Autodesk Inventor part; units mm, degrees
ref_plane "YZ Plane" through (0, 0, 0) normal (1, 0, 0) x (0, 1, 0)
ref_plane "XZ Plane" through (0, 0, 0) normal (0, 1, 0) x (-1, 0, 0)
ref_plane "XY Plane" through (0, 0, 0) normal (0, 0, 1) x (1, 0, 0)
sketch "Эскиз1" plane through (0, 0, 0) normal (0, 1, 0) x (-1, 0, 0)
  circle A0 centre (0, 0) radius 106.25
  arc A1 (-95.3337, -46.91) -> (-95.3337, 46.91) centre (-154.2365, 0) ccw
  arc A2 (95.3337, 46.91) -> (95.3337, -46.91) centre (154.2365, 0) ccw
  line L0 (-154.2365, 0) -> (154.2365, 0)
  line L1 (-95.3337, 46.91) -> (-55.3337, 46.91) construction
  line L2 (95.3337, 46.91) -> (55.3337, 46.91) construction
  point P0 (74.5593, -32.2924)
  dimension "d5" = 212.5
  dimension "d16" = 75.3
  dimension "d17" = 75.3
  dimension "d18" = 93.82
  dimension "d19" = 40
  dimension "d20" = 93.82
sketch "Эскиз2" plane through (0, 0, 0) normal (0, 0, 1) x (1, 0, 0)
  line L0 (106.25, 0) -> (-106.25, 0)
  line L1 (106.25, 0) -> (106.25, -70.1)
  line L2 (106.25, -9.1) -> (108.25, -9.1) construction
  line L3 (-149.15, 0) -> (151.15, 0)
  line L4 (106.25, -70.1) -> (104.25, -70.1)
  line L5 (104.25, -70.1) -> (104.25, -10.7208)
  line L6 (106.25, -9.1) -> (58.25, 0)
  line L7 (104.25, -10.7208) -> (58.25, -2)
  line L8 (58.25, -2) -> (58.25, 0) construction
  line L9 (50.25, 0) -> (58.25, 0)
  line L10 (50.25, 0) -> (50.25, -2)
  line L11 (50.25, -2) -> (58.25, -2)
  line L12 (0, -84.12) -> (0, 14.02)
  point P0 (0, 0)
  dimension "d0" = 70.1
  dimension "d1" = 61
  dimension "d7" = 2
  dimension "d10" = 50.25
  dimension "d11" = 8
  dimension "d34" = 2
  dimension "d35" = 1.965
revolve "Вращение1" add sketch "Эскиз2" angle 360 about axis through (0, -10, 0) along (0, 1, 0) contours L6 L1 L4 L5 L7 L11 L10 L0
chamfer "Фаска1" distance 2.5 angle 45 1 edges at (-104.25, -10.7208, 0)
extrude "Выдавливание1" cut sketch "Эскиз1" against normal through all contours L0 A2 A0 | A0 A2 L0 | A1 L0 A0 | A0 L0 A1
sketch "Эскиз3" plane through (0, 0, 0) normal (0, 1, 0) x (1, 0, 0)
  line L0 (148.75, 0) -> (-148.75, 0) construction
  line L1 (0, 148.75) -> (0, -148.75) construction
  circle A0 centre (0, 0) radius 50.25
  circle A1 centre (0, 0) radius 58.25
  circle A2 centre (0, 0) radius 54.25 construction
  circle A3 centre (-54.25, 0) radius 1.65
  circle A4 centre (0, 54.25) radius 1.65
  circle A5 centre (54.25, 0) radius 1.65
  circle A6 centre (0, -54.25) radius 1.65
  point P0 (-50.25, 0)
  point P1 (-58.25, 0)
  dimension "d23" = 8
  dimension "d24" = 4
  dimension "d25" = 3.3
  dimension "d26" = 3.3
  dimension "d27" = 3.3
  dimension "d28" = 3.3
extrude "Выдавливание2" cut sketch "Эскиз3" against normal blind 10 contours A3 | A4 | A5 | A6
sketch "Эскиз4" plane through (0, 0, 0) normal (0, 1, 0) x (1, 0, 0)
  circle A0 centre (54.25, 0) radius 1.65
  circle A1 centre (-54.25, 0) radius 1.65
  circle A2 centre (0, -54.25) radius 1.65
  circle A3 centre (0, 54.25) radius 1.65
  circle A4 centre (0, 0) radius 50.25
  circle A5 centre (0, 0) radius 58.25
chamfer "Фаска2" distance 1.4 angle 45 1 edges at (52.6, 0, 0)
equation "\"d17\" = d16"
equation "\"d20\" = d18"
equation "\"d26\" = d25"
equation "\"d27\" = d25"
equation "\"d28\" = d25"
properties part number "main_protect2"
Read the model definition and answer for the solid it produces. Units are mm, in the model's axes. A direction names the side the tool comes from. Give positions to 0.01 mm unless a question says otherwise; leave off trailing zeros. Loops run counter-clockwise (first coordinate to the right, second up) from the corner with the lowest first, then second, coordinate; pieces in that order, holes last.
Item 1: The part is cut by section A-A (y = -54). Write down the section's boundary in (x, z).
Item 2: Each of these flat-tipped pins is pushed along its axis until it touches: pin 1 Ø4 at (x, z) = (-29.5, -79) entering from +Y; pin 2 Ø5.5 at (x, z) = (0, -54.25) entering from -Y; pin 3 Ø12 at (y, z) = (-50.5, -79) entering from -X. Where does it stop, or does it pass through?
Item 3: For faces 1 (the cylindrical face through (-1.656, -40.027, -106.237)), 2 (the cylindrical face through (1.639, -41.262, -104.237)), determine the directions among +Z, -Z, +X, -X, +Y, -Y from which every point of the face is accessible in a straight line to the end or side of a thin tool.
Item 4: Find the intervals of material crossed by line 1 along Z through (x, y) = (-76, -45); line 2 along Z through (x, y) = (-77, -17.5); line 3 along X through (y, z) = (-22, 89.5), in increasing order.
Taken from the geometry:
1. outline: (-95.33, -46.91) arc R106.25 ccw to (95.33, -46.91) arc R75.3 cw to (93.97, -45.14) arc R104.25 cw to (-93.97, -45.14) arc R75.3 cw to start; (-95.33, 46.91) arc R75.3 cw to (-93.97, 45.14) arc R104.25 cw to (93.97, 45.14) arc R75.3 cw to (95.33, 46.91) arc R106.25 ccw to start
2. pin 1: stops at y = -4.56
2. pin 2: stops at y = -2
2. pin 3: stops at x = -77.2
3. face 1: -Z, +Y, -Y
3. face 2: -Y
4. line 1: z = -74.25 to -71.36, 71.36 to 74.25
4. line 2: z = -73.21 to -70.28, 70.28 to 73.21
4. line 3: x = -57.26 to -53.46, 53.46 to 57.26
